```python
from build123d import *

# Parameters (mm, degrees)
F0_R     = 6.35
F1_DEPTH = 6.35


with BuildPart() as f1:
    # F0 (on Front) → F1 (new body)
    with BuildSketch(Plane.XZ):
        with BuildLine():
            Line((-2.24177, 41.214794), (-4.592605, 37.822189))
            ThreePointArc((-4.592605, 37.822189), (-5.960153, 37.630926), (-7.319872, 37.390232))
            Line((-7.319872, 37.390232), (-10.772221, 40.018387))
            Line((-10.772221, 40.018387), (-14.868121, 38.504853))
            Line((-14.868121, 38.504853), (-16.055526, 34.551846))
            ThreePointArc((-16.055526, 34.551846), (-17.297038, 33.947349), (-18.515829, 33.298259))
            Line((-18.515829, 33.298259), (-22.611352, 34.730948))
            Line((-22.611352, 34.730948), (-26.039078, 32.02579))
            Line((-26.039078, 32.02579), (-25.946821, 27.899328))
            ThreePointArc((-25.946821, 27.899328), (-26.940768, 26.940768), (-27.899328, 25.946821))
            Line((-27.899328, 25.946821), (-32.237127, 26.043803))
            Line((-32.237127, 26.043803), (-34.661148, 22.411818))
            Line((-34.661148, 22.411818), (-33.298259, 18.515829))
            ThreePointArc((-33.298259, 18.515829), (-33.947349, 17.297038), (-34.551846, 16.055526))
            Line((-34.551846, 16.055526), (-38.707307, 14.807308))
            Line((-38.707307, 14.807308), (-39.890343, 10.604022))
            Line((-39.890343, 10.604022), (-37.390232, 7.319872))
            ThreePointArc((-37.390232, 7.319872), (-37.630926, 5.960153), (-37.822189, 4.592605))
            Line((-37.822189, 4.592605), (-41.388547, 2.121371))
            Line((-41.388547, 2.121371), (-41.214794, -2.24177))
            Line((-41.214794, -2.24177), (-37.822189, -4.592605))
            ThreePointArc((-37.822189, -4.592605), (-37.630926, -5.960153), (-37.390232, -7.319872))
            Line((-37.390232, -7.319872), (-40.018387, -10.772221))
            Line((-40.018387, -10.772221), (-38.504853, -14.868121))
            Line((-38.504853, -14.868121), (-34.551846, -16.055526))
            ThreePointArc((-34.551846, -16.055526), (-33.947349, -17.297038), (-33.298259, -18.515829))
            Line((-33.298259, -18.515829), (-34.730948, -22.611352))
            Line((-34.730948, -22.611352), (-32.02579, -26.039078))
            Line((-32.02579, -26.039078), (-27.899328, -25.946821))
            ThreePointArc((-27.899328, -25.946821), (-26.940768, -26.940768), (-25.946821, -27.899328))
            Line((-25.946821, -27.899328), (-26.043803, -32.237127))
            Line((-26.043803, -32.237127), (-22.411818, -34.661148))
            Line((-22.411818, -34.661148), (-18.515829, -33.298259))
            ThreePointArc((-18.515829, -33.298259), (-17.297038, -33.947349), (-16.055526, -34.551846))
            Line((-16.055526, -34.551846), (-14.807308, -38.707307))
            Line((-14.807308, -38.707307), (-10.604022, -39.890343))
            Line((-10.604022, -39.890343), (-7.319872, -37.390232))
            ThreePointArc((-7.319872, -37.390232), (-5.960153, -37.630926), (-4.592605, -37.822189))
            Line((-4.592605, -37.822189), (-2.121371, -41.388547))
            Line((-2.121371, -41.388547), (2.24177, -41.214794))
            Line((2.24177, -41.214794), (4.592605, -37.822189))
            ThreePointArc((4.592605, -37.822189), (5.960153, -37.630926), (7.319872, -37.390232))
            Line((7.319872, -37.390232), (10.772221, -40.018387))
            Line((10.772221, -40.018387), (14.868121, -38.504853))
            Line((14.868121, -38.504853), (16.055526, -34.551846))
            ThreePointArc((16.055526, -34.551846), (17.297038, -33.947349), (18.515829, -33.298259))
            Line((18.515829, -33.298259), (22.611352, -34.730948))
            Line((22.611352, -34.730948), (26.039078, -32.02579))
            Line((26.039078, -32.02579), (25.946821, -27.899328))
            ThreePointArc((25.946821, -27.899328), (26.940768, -26.940768), (27.899328, -25.946821))
            Line((27.899328, -25.946821), (32.237127, -26.043803))
            Line((32.237127, -26.043803), (34.661148, -22.411818))
            Line((34.661148, -22.411818), (33.298259, -18.515829))
            ThreePointArc((33.298259, -18.515829), (33.947349, -17.297038), (34.551846, -16.055526))
            Line((34.551846, -16.055526), (38.707307, -14.807308))
            Line((38.707307, -14.807308), (39.890343, -10.604022))
            Line((39.890343, -10.604022), (37.390232, -7.319872))
            ThreePointArc((37.390232, -7.319872), (37.630926, -5.960153), (37.822189, -4.592605))
            Line((37.822189, -4.592605), (41.388547, -2.121371))
            Line((41.388547, -2.121371), (41.214794, 2.24177))
            Line((41.214794, 2.24177), (37.822189, 4.592605))
            ThreePointArc((37.822189, 4.592605), (37.630926, 5.960153), (37.390232, 7.319872))
            Line((37.390232, 7.319872), (40.018387, 10.772221))
            Line((40.018387, 10.772221), (38.504853, 14.868121))
            Line((38.504853, 14.868121), (34.551846, 16.055526))
            ThreePointArc((34.551846, 16.055526), (33.947349, 17.297038), (33.298259, 18.515829))
            Line((33.298259, 18.515829), (34.730948, 22.611352))
            Line((34.730948, 22.611352), (32.02579, 26.039078))
            Line((32.02579, 26.039078), (27.899328, 25.946821))
            ThreePointArc((27.899328, 25.946821), (26.940768, 26.940768), (25.946821, 27.899328))
            Line((25.946821, 27.899328), (26.043803, 32.237127))
            Line((26.043803, 32.237127), (22.411818, 34.661148))
            Line((22.411818, 34.661148), (18.515829, 33.298259))
            ThreePointArc((18.515829, 33.298259), (17.297038, 33.947349), (16.055526, 34.551846))
            Line((16.055526, 34.551846), (14.807308, 38.707307))
            Line((14.807308, 38.707307), (10.604022, 39.890343))
            Line((10.604022, 39.890343), (7.319872, 37.390232))
            ThreePointArc((7.319872, 37.390232), (5.960153, 37.630926), (4.592605, 37.822189))
            Line((4.592605, 37.822189), (2.121387, 41.388558))
            Line((2.121387, 41.388558), (-2.24177, 41.214794))
        make_face()
        Circle(F0_R, mode=Mode.SUBTRACT)
    extrude(amount=F1_DEPTH)


solid = f1.part
```
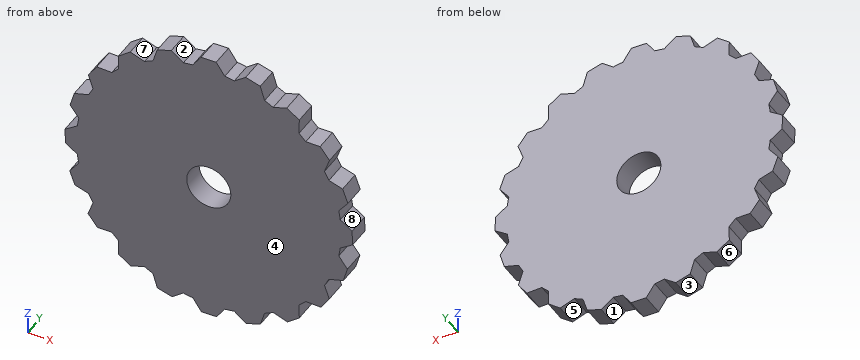
The listing builds one solid part. Answer for the finished solid, in the listing's coordinates (mm). Face numbers are marked on the shaded views. A direction names the side the tool comes from. Coordinates: 2 decimals unless noted, no trailing zeros. Write each loop counter-clockwise with the first axis right and the second up, starting at its lowest first coordinate (ties: lowest second). Pieces come first, ordered by that corner, then holes. Notation, with made-up numbers: (-25, -14.5) - (0, -14.5) arc R16 cw to (0, -3.5) - close; hole circle Ø10 at (24, -9). An arc over 180 degrees is marked (long way). Return JSON: item names as keys, results as strings. Group by question number.
Q1. Which of the six approach directions +Z, -Z, +X, -X, +Y, -Y give full straight-line access (tool end or side, diameter ignored) to the marked faces 5, 6, 7 and 8?
Q2. Flat-ended cylindrical pins translate along their axes: pin 1 Ø2 at (y, z) = (-3.5, -14.5) entering from +X; pin 2 Ø1.5 at (y, z) = (-4, 6) entering from +X. Find the tip coordinate at first contact, or state that the pin passes through.
Q3. The part is cut by section C-C on z = -13. Write down the section's boundary in (x, y).
Q4. For a pull along X with two mould halves and no side action, classify the marked faces 1, 2, 3 and 4 as +X half, -X half, draft (parallel to the pull), parting line (faces both ways), or undercut.
Q5. Find the intervals of material crossed by line 1 along X through (y, z) = (-6, -4.5); line 2 along Z through (x, y) = (0, -4); line 3 along Z through (x, y) = (-32, -3.75), in increasing order. Write a range as [from, to].
Q6. The part is cut by section B-B on z = 0. Write down the section's boundary in (x, y).
Q7. The part is cut by section A-A on x = 0. Write down the section's boundary in (y, z).
Evaluation:
{
 "1": {"face 5": "-Z, +Y, -Y", "face 6": "-Z, -X, +Y, -Y", "face 7": "+Z, +Y, -Y", "face 8": "+X, +Y, -Y"},
 "2": {"pin 1": "stops at x = 39.08", "pin 2": "stops at x = 37.74"},
 "3": {"outline": "(-39.2, -6.35) - (39.22, -6.35) - (39.22, 0) - (-39.2, 0) - close"},
 "4": {"face 1": "undercut", "face 2": "undercut", "face 3": "-X half", "face 4": "draft"},
 "5": {"line 1": "x = [-37.96, -4.48], [4.48, 37.96]", "line 2": "z = [-41.3, -6.35], [6.35, 41.3]", "line 3": "z = [-26.04, 26.04]"},
 "6": {"outline": "(-41.3, -6.35) - (-6.35, -6.35) - (-6.35, 0) - (-41.3, 0) - close; (6.35, -6.35) - (41.3, -6.35) - (41.3, 0) - (6.35, 0) - close"},
 "7": {"outline": "(-6.35, -41.3) - (0, -41.3) - (0, -6.35) - (-6.35, -6.35) - close; (-6.35, 6.35) - (0, 6.35) - (0, 41.3) - (-6.35, 41.3) - close"}
}
